Here's how the part is built. I have some questions about the finished solid (model axes, mm). A direction names the side the tool comes from. Give positions to 0.01 mm unless a question says otherwise; leave off trailing zeros. Loops run counter-clockwise (first coordinate to the right, second up) from the corner with the lowest first, then second, coordinate; pieces in that order, holes last. Notation, with made-up numbers: (-12, -18) - (46, -18) arc R24 ccw to (46, 7) - close; hole circle Ø10 at (20, 56.25). An arc over 180 degrees is marked (long way). Return JSON: item names as keys, results as strings. Group by question number.
(1) If we section it at C-C (z = 1.8): Please give me the cut outline in (x, y).
(2) If we mould it in two halves opening along X, with no side actions, what happens to faces 3 (the cylindrical face through (-14, 0, 2)), 4 (the flat face through (21, 0, 2)), 5 (the flat face through (0, 7, 4))? For each: released by +X, released by -X, zero draft, split by the parting line, or undercut.
(3) I need wall thicknesses on probe 1 along X at (y, z) = (-7.5, 0.6); probe 2 along Y at (x, z) = (3.5, 1.6); probe 3 along Y at (x, z) = (-18.5, 0.2). Which ranges of each line are inside material? Lowest first, please. Write a range as [from, to].
(4) If we section it at B-B (x = -2.5): Please give me the cut outline in (y, z).
(5) On a 3-axis mill with a long thin cutter (end or side, diameter ignored), from which of +Z, -Z, +X, -X, +Y, -Y can I reach the whole of each face in a straight line? I mean faces 1 (the flat face through (0, 7, 0)), 2 (the flat face through (0, 4.75, 2)). Say none if no direction works.
(6) If we section it at A-A (y = 0): Please give me the cut outline in (x, z).
```python
from build123d import *

# Parameters (mm, degrees)
SKETCH1_W           = 42
SKETCH1_H           = 20
SKETCH1_R           = 1.5
BOSS_EXTRUDE1_DEPTH = 4


with BuildPart() as part:
    # Sketch1 → Boss-Extrude1 (new body)
    with BuildSketch(Plane.XY):
        Rectangle(SKETCH1_W, SKETCH1_H)
        with Locations((-18.559305938, -7.559305938)):
            Circle(SKETCH1_R, mode=Mode.SUBTRACT)
        with Locations(Location((-18.559305938, 7.559305938, 0), (0, 0, 180))):
            Circle(SKETCH1_R, mode=Mode.SUBTRACT)
        with BuildLine():
            Line((-9.25, 4.75), (10.25, 4.75))
            ThreePointArc((10.25, 4.75), (15, 0), (10.25, -4.75))
            Line((10.25, -4.75), (-9.25, -4.75))
            ThreePointArc((-9.25, -4.75), (-14, 0), (-9.25, 4.75))
        make_face(mode=Mode.SUBTRACT)
    extrude(amount=BOSS_EXTRUDE1_DEPTH)


solid = part.part
```
Values:
{
 "1": {"outline": "(-21, -10) - (21, -10) - (21, 10) - (-21, 10) - close; hole circle Ø3 at (-18.56, -7.56); hole circle Ø3 at (-18.56, 7.56); hole (-9.25, -4.75) - (10.25, -4.75) arc R4.75 ccw to (10.25, 4.75) - (-9.25, 4.75) arc R4.75 ccw to start"},
 "2": {"face 3": "undercut", "face 4": "released by +X", "face 5": "zero draft"},
 "3": {"probe 1": "[-21, -20.06], [-17.06, 21]", "probe 2": "[-10, -4.75], [4.75, 10]", "probe 3": "[-10, -9.06], [-6.06, 6.06], [9.06, 10]"},
 "4": {"outline": "(-10, 0) - (-4.75, 0) - (-4.75, 4) - (-10, 4) - close; (4.75, 0) - (10, 0) - (10, 4) - (4.75, 4) - close"},
 "5": {"face 1": "-Z, +X, -X, +Y, -Y", "face 2": "+Z, -Z"},
 "6": {"outline": "(-21, 0) - (-14, 0) - (-14, 4) - (-21, 4) - close; (15, 0) - (21, 0) - (21, 4) - (15, 4) - close"}
}
